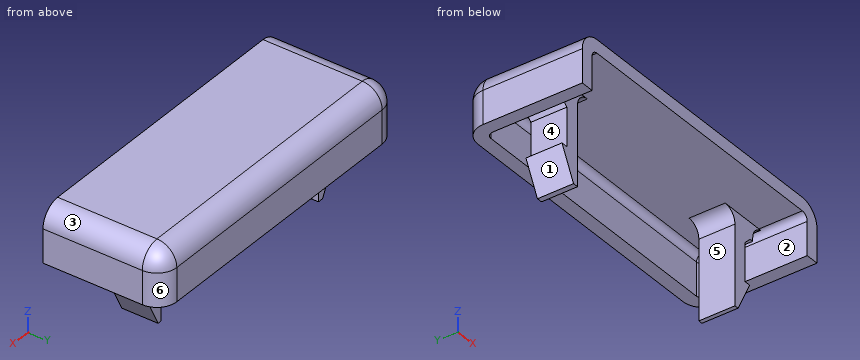
from build123d import *

# Parameters (mm, degrees)
F0_W         = 48
F0_H         = 8.0539090559
F1_DEPTH     = 18
F2_R         = 3
F3_T         = -2
F4_W         = 3.6368723959
F4_H         = 5.4553076625
F5_DEPTH     = 8
F6_W         = 3.8294224069
F6_H         = 5.4512945935
F7_DEPTH     = 8
F8_W         = 2.2997260094
F8_H         = 6.8176840032
F9_DEPTH     = 13.4
F8_W_2       = 2.9408568516
F11_T1_DEPTH = 36.529241079
F12_T1_DEPTH = 36.5332541479
F13_T1_DEPTH = 5.4512945935
F13_T3_DEPTH = 5.4553076625
F14_SIZE     = 1


# Not quite as in the source:
# - a fillet or chamfer that OpenCascade refuses, or shapes differently, is made with other operations: its cross-section is extruded or revolved along the edge and cut away or added


with BuildPart() as f1:
    # F0 (on Front) → F1 (new body)
    with BuildSketch(Plane.XZ):
        with Locations((7.3680209219, 4.0269545279)):
            Rectangle(F0_W, F0_H)
    extrude(amount=-F1_DEPTH)

    # F2
    f2_edges = [f1.edges().sort_by_distance(p)[0] for p in [
        (7.368021, 18, 8.053909),
        (-16.631979, 9, 8.053909),
        (31.368021, 9, 8.053909),
        (-16.631979, 18, 4.026955),
        (31.368021, 18, 4.026955),
    ]]
    fillet(f2_edges, radius=F2_R)

    # F3
    f3_openings = [f1.faces().sort_by_distance(p)[0] for p in [
        (7.368021, 0, 3.993074),
        (7.368021, 8.962591, 0),
    ]]
    offset(amount=F3_T, openings=f3_openings)

    # F4 (on Top) → F5 (join, symmetric)
    with BuildSketch(Plane.XY):
        with Locations((25.2722883597, 9.2779155821)):
            Rectangle(F4_W, F4_H)
    extrude(amount=F5_DEPTH, both=True)

    # F6 (on Top) → F7 (join, symmetric)
    with BuildSketch(Plane.XY):
        with Locations((-10.3424843401, 9.4998679124)):
            Rectangle(F6_W, F6_H)
    extrude(amount=F7_DEPTH, both=True)


with BuildPart() as f9:
    # F8 (on Front) → F9 (new body)
    with BuildSketch(Plane.XZ):
        with Locations((26.7013879493, 0.1128966487)):
            Rectangle(F8_W, F8_H)
    extrude(amount=-F9_DEPTH)


with BuildPart() as f9b:
    # F8 (on Front) → F9, piece 2 (new body)
    with BuildSketch(Plane.XZ):
        with Locations((-12.0930257253, 0.1128966487)):
            Rectangle(F8_W_2, F8_H)
    extrude(amount=-F9_DEPTH)


with BuildPart() as f1_1:
    add(f1.part)

    # F10: cut F9, F9b
    add(f9.part, mode=Mode.SUBTRACT)
    add(f9b.part, mode=Mode.SUBTRACT)

    # F11: chamfer of 6 x 3 on 1 edges, made by hand

    # F11_s2 → F11_t1 (cut)
    with BuildSketch(Plane.XZ.offset(-27.7644884519)):
        Polygon((-12.2571955435, -2), (-9.2571955435, -8), (-12.2571955435, -8), align=None)
    extrude(amount=F11_T1_DEPTH, mode=Mode.SUBTRACT)

    # F12: chamfer of 3 x 6 on 1 edges, made by hand

    # F12_s2 → F12_t1 (cut)
    with BuildSketch(Plane.XZ.offset(-27.544542656)):
        Polygon((27.0907245576, -2), (24.0907245576, -8), (27.0907245576, -8), align=None)
    extrude(amount=F12_T1_DEPTH, mode=Mode.SUBTRACT)

    # F13: fillet of radius 2 on 4 edges, made by hand

    # F13_s2 → F13_t1 (join)
    with BuildSketch(Plane.XZ.offset(-12.2255152091)):
        with BuildLine():
            ThreePointArc((-6.4277731366, 6.0539090559), (-7.841986699, 5.4681226183), (-8.4277731366, 4.0539090559))
            Line((-8.4277731366, 4.0539090559), (-8.4677731366, 4.0539090559))
            Line((-8.4677731366, 4.0539090559), (-8.4677731366, 6.0939090559))
            Line((-8.4677731366, 6.0939090559), (-6.4277731366, 6.0939090559))
            Line((-6.4277731366, 6.0939090559), (-6.4277731366, 6.0539090559))
        make_face()
        with BuildLine():
            ThreePointArc((-14.2571955435, 6.0539090559), (-12.8429819811, 5.4681226183), (-12.2571955435, 4.0539090559))
            Line((-12.2571955435, 4.0539090559), (-12.2171955435, 4.0539090559))
            Line((-12.2171955435, 4.0539090559), (-12.2171955435, 6.0939090559))
            Line((-12.2171955435, 6.0939090559), (-14.2571955435, 6.0939090559))
            Line((-14.2571955435, 6.0939090559), (-14.2571955435, 6.0539090559))
        make_face()
    extrude(amount=F13_T1_DEPTH)

    # F13_s4 → F13_t3 (join)
    with BuildSketch(Plane.XZ.offset(-12.0055694133)):
        with BuildLine():
            ThreePointArc((21.4538521618, 6.0539090559), (22.8680657241, 5.4681226183), (23.4538521618, 4.0539090559))
            Line((23.4538521618, 4.0539090559), (23.4938521618, 4.0539090559))
            Line((23.4938521618, 4.0539090559), (23.4938521618, 6.0939090559))
            Line((23.4938521618, 6.0939090559), (21.4538521618, 6.0939090559))
            Line((21.4538521618, 6.0939090559), (21.4538521618, 6.0539090559))
        make_face()
        with BuildLine():
            ThreePointArc((29.0907245576, 6.0539090559), (27.6765109953, 5.4681226183), (27.0907245576, 4.0539090559))
            Line((27.0907245576, 4.0539090559), (27.0507245576, 4.0539090559))
            Line((27.0507245576, 4.0539090559), (27.0507245576, 6.0939090559))
            Line((27.0507245576, 6.0939090559), (29.0907245576, 6.0939090559))
            Line((29.0907245576, 6.0939090559), (29.0907245576, 6.0539090559))
        make_face()
    extrude(amount=F13_T3_DEPTH)

    # F14
    f14_edges = [f1_1.edges().sort_by_distance(p)[0] for p in [
        (25.551525, 9.277916, 3.521739),
        (-10.622597, 9.499868, 3.521739),
    ]]
    chamfer(f14_edges, length=F14_SIZE)


solid = f1_1.part
Verification items for the finished model (mm, model axes). Face numbers are marked on the shaded views. A direction names the side the tool comes from. Coordinates: 2 decimals unless noted, no trailing zeros. Write each loop counter-clockwise with the first axis right and the second up, starting at its lowest first coordinate (ties: lowest second). Pieces come first, ordered by that corner, then holes. Notation, with made-up numbers: (51, 7.5) -> (71, 7.5) arc R30 ccw to (71, 46.5) -> close; hole circle Ø8 at (-31, 24.5). An arc over 180 degrees is marked (long way). One line per item, written item: value. Start each with the question number.
Q1. Thickness scan on L1, parallel to X at y = 8.25, z = 1.5; L2, parallel to X at y = 7.25, z = 4; L3, parallel to Y at x = -10, z = 1. Record the ranges inside material, lowest first. Write a range as from..to.
Q2. Mould release check, pull along X, two halves, no side actions. Record for the marked faces 1, 2 and 3: pulls with the +X half, pulls with the -X half, needs draft (parallel to the pull), parting line crosses it, or undercut.
Q3. Go/stop test with flat-tipped pins: P1, Ø1.6, axis at y = 10.5, z = -2, coming from the +X side; P2, Ø1.6, axis at y = 10.5, z = -4, coming from the +X side; P3, Ø4.5, axis at x = 11.5, y = 9.5, coming from the -Z side; P4, Ø1, axis at y = 5, z = -4, coming from the -X side. Record where each tip stops, or that it passes through.
Q4. Cross-section at B-B on x = 26. Enter the section's corners in (y, z), and give its area (3 significant figures).
Q5. Cross-section at A-A on z = -2. Enter the section's corners in (x, y).
Q6. Access from +Z, -Z, +X, -X, +Y, -Y to the whole of each face (thin tool, end or side, straight path). Record for the marked faces 4, 5 and 6.
Q7. Cross-section at D-D on z = 0.5. Enter the section's corners in (x, y), and give its area (3 significant figures).
Checked values:
1. L1: x = -16.63..-14.63, -10.62..-8.43, 23.45..25.55, 29.37..31.37
1. L2: x = -16.63..-14.63, -12.26..-8.43, 23.45..27.09, 29.37..31.37
1. L3: y = 6.77..12.23, 16..18
2. face 1: pulls with the -X half
2. face 2: undercut
2. face 3: pulls with the +X half
3. P1: stops at x = 25.55
3. P2: stops at x = 26.44
3. P3: stops at z = 6.05
3. P4: passes through
4. outline: (0, 6.05) -> (6.55, 6.05) -> (6.55, 2.97) -> (12.01, 2.97) -> (12.01, 6.05) -> (15, 6.05) arc R1 cw to (16, 5.05) -> (16, 0) -> (18, 0) -> (18, 5.05) arc R3 ccw to (15, 8.05) -> (0, 8.05) -> close; (6.55, -4.18) -> (12.01, -4.18) -> (12.01, -3.3) -> (6.55, -3.3) -> close
4. area: 68.0 mm²
5. outline: (-10.62, 6.77) -> (-8.43, 6.77) -> (-8.43, 12.23) -> (-10.62, 12.23) -> close; (23.45, 6.55) -> (25.55, 6.55) -> (25.55, 12.01) -> (23.45, 12.01) -> close
6. face 4: -Y
6. face 5: -Z, -Y
6. face 6: +Z, -Z, +X, +Y
7. outline: (-16.63, 0) -> (-14.63, 0) -> (-14.63, 15) arc R1 cw to (-13.63, 16) -> (28.37, 16) arc R1 cw to (29.37, 15) -> (29.37, 0) -> (31.37, 0) -> (31.37, 15) arc R3 ccw to (28.37, 18) -> (-13.63, 18) arc R3 ccw to (-16.63, 15) -> close; (-10.62, 6.77) -> (-8.43, 6.77) -> (-8.43, 12.23) -> (-10.62, 12.23) -> close; (23.45, 6.55) -> (25.55, 6.55) -> (25.55, 12.01) -> (23.45, 12.01) -> close
7. area: 180 mm²
